Read the model definition and answer for the solid it produces. Units are mm, in the model's axes. Face numbers are marked on the shaded views. A direction names the side the tool comes from. Coordinates: 2 decimals unless noted, no trailing zeros. Write each loop counter-clockwise with the first axis right and the second up, starting at its lowest first coordinate (ties: lowest second). Pieces come first, ordered by that corner, then holes.
Item 1: Section D-D (x = -200.5) is taken. Give the vertices of the cut face in (y, z) (1 decimal).
Item 2: Section B-B (z = 18) is taken. Give the vertices of the cut face in (x, y), then the cut area to 3 significant figures.
Item 3: Section C-C (y = -19) is taken. Give the vertices of the cut face in (x, z) (3 decimals).
Item 4: Section A-A (y = 76.5) is taken. State how many separate pieces and enclosed holes the cut face has, then the cut area to 3 significant figures.
Item 5: A tool of negligible diameter and unlimited length cuts with its end or side. For the marked faces 1 and 2, from which of +Z, -Z, +X, -X, +Y, -Y can it reach the whole face along a straight path? Write none if from no direction.
Item 6: Determine the mould class of the marked faces 3, 4 and 5 for opening direction X: released by +X, released by -X, zero draft, split by the parting line, or undercut.
Item 7: Each of these flat-tipped pins is pushed along its axis until it touches: P1, Ø5, axis at x = 169.51, y = 43.15, coming from the -Z side (3 decimals); P2, Ø2.5, axis at y = -64.5, z = 61.5, coming from the -X side; P3, Ø3, axis at y = -95, z = 34.5, coming from the -X side; P4, Ø7, axis at x = -90.84, y = 43.15, coming from the +Z side. Where does it stop, or does it pass through?
Item 8: Straight lines are drawn through the part: probe 1 along X at (y, z) = (-113.5, -14) (3 decimals); probe 2 along Z at (x, y) = (118.5, -47) (3 decimals); probe 3 along Y at (x, z) = (-121.5, -6) (3 decimals). For each, find the intervals that lie inside material, in ascending order.
from build123d import *

# Parameters (mm, degrees)
SKETCH1_W               = 647.7
SKETCH1_H               = 402.59
BOSS_EXTRUDE1_DEPTH     = 63.5
CHAMFER1_SIZE           = 63.5
CHAMFER2_SIZE           = 63.5
SKETCH3_W               = 647.7
SKETCH3_H               = 402.59
BOSS_EXTRUDE2_DEPTH     = 17.78
SHELL1_T                = -3.175
SKETCH4_W               = 641.35
SKETCH4_H               = 3.175
CUT_EXTRUDE1_DEPTH      = 17.78
CUT_EXTRUDE3_DEPTH      = 390.878106496
CUT_EXTRUDE3_DEPTH_BACK = 390.878106496
SKETCH2_R               = 2.25


with BuildPart() as part:
    # Sketch1 → Boss-Extrude1 (new body)
    with BuildSketch(Plane.XY):
        Rectangle(SKETCH1_W, SKETCH1_H)
    extrude(amount=BOSS_EXTRUDE1_DEPTH)

    # Chamfer1
    chamfer1_edges = [part.edges().sort_by_distance(p)[0] for p in [
        (0, 201.295, 63.5),
        (0, -201.295, 63.5),
    ]]
    chamfer(chamfer1_edges, length=CHAMFER1_SIZE - 0.0001)  # a hair under: the kernel refuses the full size

    # Chamfer2
    chamfer2_edges = [part.edges().sort_by_distance(p)[0] for p in [
        (-323.85, 0, 63.5),
        (323.85, 0, 63.5),
    ]]
    chamfer(chamfer2_edges, length=CHAMFER2_SIZE - 0.0001)  # a hair under: the kernel refuses the full size

    # Sketch3 → Boss-Extrude2 (add)
    with BuildSketch(Plane.XY):
        Rectangle(SKETCH3_W, SKETCH3_H)
    extrude(amount=-BOSS_EXTRUDE2_DEPTH)

    # Shell1
    shell1_openings = [part.faces().sort_by_distance(p)[0] for p in [
        (0, 0, -17.78),
    ]]
    offset(amount=SHELL1_T, openings=shell1_openings, kind=Kind.INTERSECTION)

    # Sketch4 → Cut-Extrude1 (cut)
    with BuildSketch(Plane(origin=(0, 0, -17.78), x_dir=(-1, 0, 0), z_dir=(0, 0, -1))):
        with Locations((0, 199.7075)):
            Rectangle(SKETCH4_W, SKETCH4_H)
    extrude(amount=-CUT_EXTRUDE1_DEPTH, mode=Mode.SUBTRACT)

    # Sketch2 → Cut-Extrude3 (cut, two sides: drawn at the far end of the back side and taken through both)
    with BuildSketch(Plane.XY.offset(63.5).offset(-CUT_EXTRUDE3_DEPTH_BACK)):
        with BuildLine():
            Line((-37.107499953, 53.0225), (-37.107499953, 84.7725))
            ThreePointArc((-37.107499953, 84.7725), (-41.723671365, 92.261328635), (-49.2125, 96.877500047))
            Line((-49.2125, 96.877500047), (-80.9625, 96.877500047))
            ThreePointArc((-80.9625, 96.877500047), (-88.451328635, 92.261328635), (-93.067500047, 84.7725))
            Line((-93.067500047, 84.7725), (-93.067500047, 53.0225))
            ThreePointArc((-93.067500047, 53.0225), (-88.451328635, 45.533671365), (-80.9625, 40.917499953))
            Line((-80.9625, 40.917499953), (-49.2125, 40.917499953))
            ThreePointArc((-49.2125, 40.917499953), (-41.723671365, 45.533671365), (-37.107499953, 53.0225))
        make_face()
        with Locations((-221.012500062, 43.147499938)):
            Circle(SKETCH2_R)
        with Locations((-169.512499938, 43.147499938)):
            Circle(SKETCH2_R)
        with Locations((-39.337499938, 94.647500062)):
            Circle(SKETCH2_R)
        with Locations((-90.837500062, 43.147499938)):
            Circle(SKETCH2_R)
        with Locations((-39.337499938, 43.147499938)):
            Circle(SKETCH2_R)
        with BuildLine():
            ThreePointArc((80.9625, 96.877500047), (88.451328635, 92.261328635), (93.067500047, 84.7725))
            Line((93.067500047, 84.7725), (93.067500047, 53.0225))
            ThreePointArc((93.067500047, 53.0225), (88.451328635, 45.533671365), (80.9625, 40.917499953))
            Line((80.9625, 40.917499953), (49.2125, 40.917499953))
            ThreePointArc((49.2125, 40.917499953), (41.723671365, 45.533671365), (37.107499953, 53.0225))
            Line((37.107499953, 53.0225), (37.107499953, 84.7725))
            ThreePointArc((37.107499953, 84.7725), (41.723671365, 92.261328635), (49.2125, 96.877500047))
            Line((49.2125, 96.877500047), (80.9625, 96.877500047))
        make_face()
        with BuildLine():
            Line((223.242500047, 53.0225), (223.242500047, 84.7725))
            ThreePointArc((223.242500047, 84.7725), (218.626328635, 92.261328635), (211.1375, 96.877500047))
            Line((211.1375, 96.877500047), (179.3875, 96.877500047))
            ThreePointArc((179.3875, 96.877500047), (171.898671365, 92.261328635), (167.282499953, 84.7725))
            Line((167.282499953, 84.7725), (167.282499953, 53.0225))
            ThreePointArc((167.282499953, 53.0225), (171.898671365, 45.533671365), (179.3875, 40.917499953))
            Line((179.3875, 40.917499953), (211.1375, 40.917499953))
            ThreePointArc((211.1375, 40.917499953), (218.626328635, 45.533671365), (223.242500047, 53.0225))
        make_face()
        with BuildLine():
            Line((-223.242500047, -53.0225), (-223.242500047, -84.7725))
            ThreePointArc((-223.242500047, -84.7725), (-218.626328635, -92.261328635), (-211.1375, -96.877500047))
            Line((-211.1375, -96.877500047), (-179.3875, -96.877500047))
            ThreePointArc((-179.3875, -96.877500047), (-171.898671365, -92.261328635), (-167.282499953, -84.7725))
            Line((-167.282499953, -84.7725), (-167.282499953, -53.0225))
            ThreePointArc((-167.282499953, -53.0225), (-171.898671365, -45.533671365), (-179.3875, -40.917499953))
            Line((-179.3875, -40.917499953), (-211.1375, -40.917499953))
            ThreePointArc((-211.1375, -40.917499953), (-218.626328635, -45.533671365), (-223.242500047, -53.0225))
        make_face()
        with BuildLine():
            ThreePointArc((-80.9625, -96.877500047), (-88.451328635, -92.261328635), (-93.067500047, -84.7725))
            Line((-93.067500047, -84.7725), (-93.067500047, -53.0225))
            ThreePointArc((-93.067500047, -53.0225), (-88.451328635, -45.533671365), (-80.9625, -40.917499953))
            Line((-80.9625, -40.917499953), (-49.2125, -40.917499953))
            ThreePointArc((-49.2125, -40.917499953), (-41.723671365, -45.533671365), (-37.107499953, -53.0225))
            Line((-37.107499953, -53.0225), (-37.107499953, -84.7725))
            ThreePointArc((-37.107499953, -84.7725), (-41.723671365, -92.261328635), (-49.2125, -96.877500047))
            Line((-49.2125, -96.877500047), (-80.9625, -96.877500047))
        make_face()
        with BuildLine():
            Line((37.107499953, -53.0225), (37.107499953, -84.7725))
            ThreePointArc((37.107499953, -84.7725), (41.723671365, -92.261328635), (49.2125, -96.877500047))
            Line((49.2125, -96.877500047), (80.9625, -96.877500047))
            ThreePointArc((80.9625, -96.877500047), (88.451328635, -92.261328635), (93.067500047, -84.7725))
            Line((93.067500047, -84.7725), (93.067500047, -53.0225))
            ThreePointArc((93.067500047, -53.0225), (88.451328635, -45.533671365), (80.9625, -40.917499953))
            Line((80.9625, -40.917499953), (49.2125, -40.917499953))
            ThreePointArc((49.2125, -40.917499953), (41.723671365, -45.533671365), (37.107499953, -53.0225))
        make_face()
        with BuildLine():
            ThreePointArc((179.3875, -96.877500047), (171.898671365, -92.261328635), (167.282499953, -84.7725))
            Line((167.282499953, -84.7725), (167.282499953, -53.0225))
            ThreePointArc((167.282499953, -53.0225), (171.898671365, -45.533671365), (179.3875, -40.917499953))
            Line((179.3875, -40.917499953), (211.1375, -40.917499953))
            ThreePointArc((211.1375, -40.917499953), (218.626328635, -45.533671365), (223.242500047, -53.0225))
            Line((223.242500047, -53.0225), (223.242500047, -84.7725))
            ThreePointArc((223.242500047, -84.7725), (218.626328635, -92.261328635), (211.1375, -96.877500047))
            Line((211.1375, -96.877500047), (179.3875, -96.877500047))
        make_face()
        with Locations((39.337499938, 94.647500062)):
            Circle(SKETCH2_R)
        with Locations((90.837500062, 94.647500062)):
            Circle(SKETCH2_R)
        with Locations((90.837500062, 43.147499938)):
            Circle(SKETCH2_R)
        with Locations((-221.012500062, -43.147499938)):
            Circle(SKETCH2_R)
        with Locations((-169.512499938, -43.147499938)):
            Circle(SKETCH2_R)
        with Locations((-169.512499938, -94.647500062)):
            Circle(SKETCH2_R)
        with Locations((-90.837500062, -43.147499938)):
            Circle(SKETCH2_R)
        with Locations((-39.337499938, -43.147499938)):
            Circle(SKETCH2_R)
        with Locations((-90.837500062, -94.647500062)):
            Circle(SKETCH2_R)
        with Locations((39.337499938, -43.147499938)):
            Circle(SKETCH2_R)
        with Locations((39.337499938, -94.647500062)):
            Circle(SKETCH2_R)
        with Locations((90.837500062, -43.147499938)):
            Circle(SKETCH2_R)
        with Locations((90.837500062, -94.647500062)):
            Circle(SKETCH2_R)
        with Locations((169.512499938, -43.147499938)):
            Circle(SKETCH2_R)
        with Locations((221.012500062, -43.147499938)):
            Circle(SKETCH2_R)
        with Locations((169.512499938, -94.647500062)):
            Circle(SKETCH2_R)
        with Locations((221.012500062, -94.647500062)):
            Circle(SKETCH2_R)
        with BuildLine():
            ThreePointArc((-223.242500047, 84.7725), (-218.626328635, 92.261328635), (-211.1375, 96.877500047))
            Line((-211.1375, 96.877500047), (-179.3875, 96.877500047))
            ThreePointArc((-179.3875, 96.877500047), (-171.898671365, 92.261328635), (-167.282499953, 84.7725))
            Line((-167.282499953, 84.7725), (-167.282499953, 53.0225))
            ThreePointArc((-167.282499953, 53.0225), (-171.898671365, 45.533671365), (-179.3875, 40.917499953))
            Line((-179.3875, 40.917499953), (-211.1375, 40.917499953))
            ThreePointArc((-211.1375, 40.917499953), (-218.626328635, 45.533671365), (-223.242500047, 53.0225))
            Line((-223.242500047, 53.0225), (-223.242500047, 84.7725))
        make_face()
        with Locations((-221.012500062, 94.647500062)):
            Circle(SKETCH2_R)
        with Locations((-169.512499938, 94.647500062)):
            Circle(SKETCH2_R)
        with Locations((-90.837500062, 94.647500062)):
            Circle(SKETCH2_R)
        with Locations((39.337499938, 43.147499938)):
            Circle(SKETCH2_R)
        with Locations((169.512499938, 94.647500062)):
            Circle(SKETCH2_R)
        with Locations((169.512499938, 43.147499938)):
            Circle(SKETCH2_R)
        with Locations((221.012500062, 94.647500062)):
            Circle(SKETCH2_R)
        with Locations((221.012500062, 43.147499938)):
            Circle(SKETCH2_R)
        with Locations((-221.012500062, -94.647500062)):
            Circle(SKETCH2_R)
        with Locations((-39.337499938, -94.647500062)):
            Circle(SKETCH2_R)
    extrude(amount=CUT_EXTRUDE3_DEPTH + CUT_EXTRUDE3_DEPTH_BACK, mode=Mode.SUBTRACT)


solid = part.part
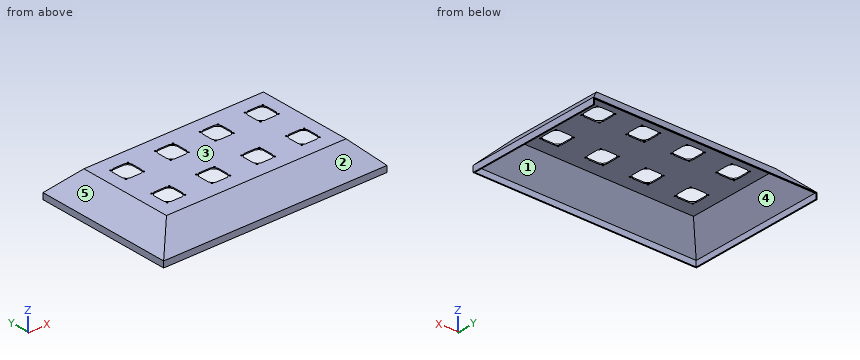
Established:
1. outline: (-201.3, -17.8) - (-198.1, -17.8) - (-198.1, -1.3) - (-136.5, 60.3) - (-96.9, 60.3) - (-96.9, 63.5) - (-137.8, 63.5) - (-201.3, 0) - close; (-40.9, 60.3) - (40.9, 60.3) - (40.9, 63.5) - (-40.9, 63.5) - close; (96.9, 60.3) - (136.5, 60.3) - (198.1, -1.3) - (198.1, 0) - (201.3, 0) - (137.8, 63.5) - (96.9, 63.5) - close
2. outline: (-305.85, -183.3) - (305.85, -183.3) - (305.85, 183.3) - (-305.85, 183.3) - close; hole (-301.36, -178.8) - (301.36, -178.8) - (301.36, 178.8) - (-301.36, 178.8) - close
2. area: 8,700 mm2
3. outline: (-323.85, -17.78) - (-320.675, -17.78) - (-320.675, -1.315) - (-259.035, 60.325) - (259.035, 60.325) - (320.675, -1.315) - (320.675, -17.78) - (323.85, -17.78) - (323.85, 0) - (260.35, 63.5) - (-260.35, 63.5) - (-323.85, 0) - close
4. separate pieces: 5
4. enclosed holes: 0
4. area: 1,610 mm2
5. face 1: -Z
5. face 2: +Z, +X, -X, -Y
6. face 3: zero draft
6. face 4: undercut
6. face 5: released by -X
7. P1: stops at z = 60.325
7. P2: stops at x = -263.6
7. P3: stops at x = -290.85
7. P4: stops at z = 63.5
8. probe 1: x = -323.85 to -320.675, 320.675 to 323.85
8. probe 2: z = 60.325 to 63.5
8. probe 3: y = -201.295 to -198.12
